Verification items for the finished model (mm, model axes). A direction names the side the tool comes from. Give positions to 0.01 mm unless a question says otherwise; leave off trailing zeros. Loops run counter-clockwise (first coordinate to the right, second up) from the corner with the lowest first, then second, coordinate; pieces in that order, holes last. Notation, with made-up numbers: M 20,77.25 L 78,77.25 A25 ccw 78,89.25 Z; hole C 48,57 d8. An arc over 180 degrees is marked long. Put each result on its own line as item: value. Start each with the question number.
from build123d import *

# Parameters (mm, degrees)
F1_W     = 62
F1_H     = 112
F2_DEPTH = 5
F4_DEPTH = 5
F5_R     = 5


with BuildPart() as f2:
    # F1 (on Front) → F2 (new body)
    with BuildSketch(Plane.XZ):
        with Locations((3.447434, 3.619151)):
            Rectangle(F1_W, F1_H)
    extrude(amount=F2_DEPTH)

    # F3 (on Front) → F4 (cut)
    with BuildSketch(Plane.XZ):
        with BuildLine():
            ThreePointArc((30.516835, 32.039018), (26.895076, 40.782716), (18.151378, 44.404474))
            Line((18.151378, 44.404474), (-19.549268, 44.404474))
            ThreePointArc((-19.549268, 44.404474), (-22.423638, 43.213804), (-23.614078, 40.339338))
            Line((-23.614078, 40.339338), (-23.607969, -35.961972))
            ThreePointArc((-23.607969, -35.961972), (-19.98765, -44.70071), (-11.248622, -48.320329))
            Line((-11.248622, -48.320329), (26.451378, -48.320329))
            ThreePointArc((26.451378, -48.320329), (29.32177, -47.131374), (30.510725, -44.260982))
            Line((30.510725, -44.260982), (30.516835, 32.039018))
        make_face()
    extrude(amount=F4_DEPTH, mode=Mode.SUBTRACT)

    # F5
    f5_edges = [f2.edges().sort_by_distance(p)[0] for p in [
        (-27.552566, -2.5, 59.619151),
        (-27.552566, -2.5, -52.380849),
        (34.447434, -2.5, -52.380849),
        (34.447434, -2.5, 59.619151),
    ]]
    fillet(f5_edges, radius=F5_R)


solid = f2.part
Q1. Cross-section at A-A, the plane x = 15.5. Record the boundary of the cut face in (y, z).
Q2. Go/stop test with a flat-tipped pin: pin 1 (12 mm diameter, centred on x = 24.5, z = 35, fed in from +Y). Record where the tip stops, or that it passes through.
Q3. Cross-section at C-C, the plane y = -2.1. Record the boundary of the cut face in (x, z), then the cut area to 3 significant figures.
Q4. Release check for a two-part mould opening along Z. For faces 1 (the face through (26.991, -2.465, 40.686)), 2 (the face through (3, -2, -52.381)), 3 (the face through (29.29, -2.46, -47.16)), 4 (the face through (-27.553, -2, 3)) record: pulls with the +Z half, pulls with the -Z half, needs draft (parallel to the pull), parting line crosses it, or undercut.
Q5. Cross-section at B-B, the plane z = -13. Record the boundary of the cut face in (x, y).
Q6. Set-up check for faces 5 (the face through (-24, 0, 8)), 6 (the face through (-20.083, -2.465, -44.604)): record each of +Z, -Z, +X, -X, +Y, -Y from which the full face is reachable in a straight line by a thin tool's end or side.
Q7. Scan lines: L1, parallel to X at y = -2.4, z = 1.5; L2, parallel to Z at x = -7.5, y = -0.4; L3, parallel to Z at x = -16, y = -0.4. Record each from-to range of solid material in increasing order.
Ans:
1. outline: M -5,-52.38 L 0,-52.38 L 0,-48.32 L -5,-48.32 Z; M -5,44.4 L 0,44.4 L 0,59.62 L -5,59.62 Z
2. pin 1: stops at y = 0
3. outline: M -27.55,-47.38 A5 ccw -22.55,-52.38 L 29.45,-52.38 A5 ccw 34.45,-47.38 L 34.45,54.62 A5 ccw 29.45,59.62 L -22.55,59.62 A5 ccw -27.55,54.62 Z; hole M -23.61,-35.96 A12.36 ccw -11.25,-48.32 L 26.45,-48.32 A4.06 ccw 30.51,-44.26 L 30.52,32.04 A12.37 ccw 18.15,44.4 L -19.55,44.4 A4.06 ccw -23.61,40.34 Z
3. area: 1,980 mm^2
4. face 1: undercut
4. face 2: pulls with the -Z half
4. face 3: undercut
4. face 4: needs draft
5. outline: M -27.55,-5 L -23.61,-5 L -23.61,0 L -27.55,0 Z; M 30.51,-5 L 34.45,-5 L 34.45,0 L 30.51,0 Z
6. face 5: +Z, -Z, +X, -X, +Y
6. face 6: +Y, -Y
7. L1: x = -27.55 to -23.61, 30.51 to 34.45
7. L2: z = -52.38 to -48.32, 44.4 to 59.62
7. L3: z = -52.38 to -47.37, 44.4 to 59.62
